For this review, take the finished solid that the model builds, in its own axes (mm). A direction names the side the tool comes from. Coordinates: 2 decimals unless noted, no trailing zeros. Loops run counter-clockwise (first coordinate to the right, second up) from the corner with the lowest first, then second, coordinate; pieces in that order, holes last. Notation, with made-up numbers: (88, 51.25) -> (122, 51.25) arc R15 ccw to (122, 77.25) -> close; hole circle Ø9 at (-26.5, -3.75). An arc over 180 degrees is marked (long way). One line per item, written item: value.
from build123d import *

# Parameters (mm, degrees)
F0_W      = 60.96
F0_H      = 104.14
F1_DEPTH  = 4.1
F2_W      = 50.8
F2_H      = 38.1
F2_R      = 17.78
F2_R_2    = 7.62
F3_DEPTH  = 0.635
F4_R      = 5.08
F5_R      = 1.27
F6_DEPTH  = 3.81
F7_W      = 0.127
F7_H      = 0.635
F7_H_2    = 0.641739
F8_DEPTH  = 0.0635
F9_W      = 23.568134
F9_H      = 1.790789
F10_DEPTH = 6.35
F11_W     = 11.43
F11_H     = 1.143
F12_DEPTH = 0.381
F13_R     = 0.9525
F14_DEPTH = 5.08
F15_W     = 0.323782
F15_H     = 1.115247
F15_W_2   = 0.323781
F16_DEPTH = 0.0381


with BuildPart() as f1:
    # F0 (on Front) → F1 (new body)
    with BuildSketch(Plane.XZ):
        with Locations((3.610969, -7.489684)):
            Rectangle(F0_W, F0_H)
    extrude(amount=F1_DEPTH)

    # F2 (on face) → F3 (join)
    with BuildSketch(Plane.XZ.offset(4.1)):
        with Locations((3.610969, 19.180316)):
            Rectangle(F2_W, F2_H)
        with Locations((3.610969, -28.233618)):
            Circle(F2_R)
        with Locations((3.610969, -28.233618)):
            Circle(F2_R_2, mode=Mode.SUBTRACT)
    extrude(amount=F3_DEPTH)

    # F4
    f4_edges = [f1.edges().sort_by_distance(p)[0] for p in [
        (-26.869031, -2.05, 44.580316),
        (34.090969, -2.05, 44.580316),
        (34.090969, -2.05, -59.559684),
        (-26.869031, -2.05, -59.559684),
    ]]
    fillet(f4_edges, radius=F4_R)

    # F5 (on face) → F6 (cut)
    with BuildSketch(Plane.XY.offset(44.580316)):
        with Locations((25.835969, -8.355387)):
            Circle(F5_R)
    extrude(amount=-F6_DEPTH, mode=Mode.SUBTRACT)

    # F7 (on face) → F8 (cut)
    with BuildSketch(Plane.XY.offset(44.580316)):
        with Locations((23.406764, -8.501846)):
            Rectangle(F7_W, F7_H)
        with Locations((23.75507, -8.505765)):
            Rectangle(F7_W, F7_H_2)
    extrude(amount=-F8_DEPTH, mode=Mode.SUBTRACT)

    # F9 (on face) → F10 (cut)
    with BuildSketch(Plane(origin=(0, 0, -59.559684), x_dir=(1, 0, 0), z_dir=(0, 0, -1))):
        with Locations((4.526902, 2.315605)):
            Rectangle(F9_W, F9_H)
    extrude(amount=-F10_DEPTH, mode=Mode.SUBTRACT)

    # F11 (on face) → F12 (join)
    with BuildSketch(Plane.XY.offset(44.580316)):
        with Locations((-13.885994, -2.445143)):
            Rectangle(F11_W, F11_H)
    extrude(amount=F12_DEPTH)

    # F13 (on face) → F14 (cut)
    with BuildSketch(Plane.XY.offset(44.580316)):
        with Locations((25.083786, -2.716642)):
            Circle(F13_R)
    extrude(amount=-F14_DEPTH, mode=Mode.SUBTRACT)

    # F15 (on face) → F16 (join)
    with BuildSketch(Plane.XY.offset(44.580316)):
        with Locations((21.622912, -2.742082)):
            Rectangle(F15_W, F15_H)
        with Locations((22.481088, -2.742082)):
            Rectangle(F15_W_2, F15_H)
    extrude(amount=F16_DEPTH)


solid = f1.part
1. Insertion check: pin 1 Ø0.7 at (y, z) = (-4.5, 11) entering from +X; pin 2 Ø2 at (x, z) = (-18, -40) entering from -Y; pin 3 Ø1.4 at (y, z) = (-2, -57.5) entering from -X. Each pin has a flat end and moves straight along its axis. Give the tip position at first contact, or say it passes through.
Return value:
pin 1: stops at x = 29.01
pin 2: stops at y = -4.1
pin 3: stops at x = -26.31
2. For faces 1 (the cylindrical face through (24.877, -3.646, 42.076)), 2 (the flat face through (4, -4.1, -28)), 3 (the flat face through (4, -3.211, -56)), list the 3-axis set-ups (+Z, -Z, +X, -X, +Y, -Y) from which the entire face can be reached by the end or side of a thin tool; tool diameter is ignored.
Return value:
face 1: +Z
face 2: -Y
face 3: -Z
3. Take a section at A-A, the plane z = 14. Give the boundary of the cut face in (x, y) (3 decimals), and give its area (3 significant figures).
Return value:
outline: (-26.869, -4.1) -> (-21.789, -4.1) -> (-21.789, -4.735) -> (29.011, -4.735) -> (29.011, -4.1) -> (34.091, -4.1) -> (34.091, 0) -> (-26.869, 0) -> close
area: 282 mm2
4. Take a section at D-D, the plane x = 8. Give the boundary of the cut face in (y, z) (3 decimals), and give its area (3 significant figures).
Return value:
outline: (-4.735, -45.463) -> (-4.1, -45.463) -> (-4.1, -59.56) -> (-3.211, -59.56) -> (-3.211, -53.21) -> (-1.42, -53.21) -> (-1.42, -59.56) -> (0, -59.56) -> (0, 44.58) -> (-4.1, 44.58) -> (-4.1, 38.23) -> (-4.735, 38.23) -> (-4.735, 0.13) -> (-4.1, 0.13) -> (-4.1, -11.004) -> (-4.735, -11.004) -> (-4.735, -22.005) -> (-4.1, -22.005) -> (-4.1, -34.463) -> (-4.735, -34.463) -> close
area: 454 mm2
5. Take a section at C-C, the plane z = -22.5. Give the boundary of the cut face in (x, y) (3 decimals).
Return value:
outline: (-26.869, -4.1) -> (-13.219, -4.1) -> (-13.219, -4.735) -> (-1.408, -4.735) -> (-1.408, -4.1) -> (8.63, -4.1) -> (8.63, -4.735) -> (20.441, -4.735) -> (20.441, -4.1) -> (34.091, -4.1) -> (34.091, 0) -> (-26.869, 0) -> close
6. Take a section at B-B, the plane x = 1. Give the boundary of the cut face in (y, z) (3 decimals), and give its area (3 significant figures).
Return value:
outline: (-4.735, -45.821) -> (-4.1, -45.821) -> (-4.1, -59.56) -> (-3.211, -59.56) -> (-3.211, -53.21) -> (-1.42, -53.21) -> (-1.42, -59.56) -> (0, -59.56) -> (0, 44.58) -> (-4.1, 44.58) -> (-4.1, 38.23) -> (-4.735, 38.23) -> (-4.735, 0.13) -> (-4.1, 0.13) -> (-4.1, -10.646) -> (-4.735, -10.646) -> (-4.735, -21.075) -> (-4.1, -21.075) -> (-4.1, -35.392) -> (-4.735, -35.392) -> close
area: 453 mm2
7. To check wall thickness, follow probe 1 along Y at (x, z) = (9.5, -54); probe 2 along Z at (x, y) = (3, -1); probe 3 along Z at (x, y) = (29.5, -1.7). State the ranges of each line that lie inside material, in increasing order. Write a range as from..to.
Return value:
probe 1: y = -4.1..-3.21, -1.42..0
probe 2: z = -59.56..44.58
probe 3: z = -59.54..44.56
8. The part is to be moulded in two halves that separate along Z. For faces 4 (the cylindrical face through (32.563, -2.079, -58.111)), 5 (the flat face through (25, -3, 39.5)), 6 (the cylindrical face through (-2.436, -4.413, -32.87)), say which applies: pulls with the +Z half, pulls with the -Z half, needs draft (parallel to the pull), parting line crosses it, or undercut.
Return value:
face 4: pulls with the -Z half
face 5: pulls with the +Z half
face 6: undercut
